Could you check a few things on this model? Use its own coordinates, in mm. A direction names the side the tool comes from. Give positions to 0.01 mm unless a question says otherwise; leave off trailing zeros. Write each loop counter-clockwise with the first axis right and the second up, starting at its lowest first coordinate (ties: lowest second). Pieces come first, ordered by that corner, then holes. Notation, with made-up numbers: M -12.75,59 L 36.25,59 A31 cw 36.25,90 Z; hole C 56,-14.75 d1. An arc over 180 degrees is marked long. Answer as a JSON object with one key per item and string values. Group by question number.
```python
from build123d import *

# Parameters (mm, degrees)
SKETCH1_W           = 100
SKETCH1_H           = 65
BOSS_EXTRUDE1_DEPTH = 35
SKETCH4_W           = 60
SKETCH4_H           = 30
CUT_EXTRUDE1_DEPTH  = 6
SKETCH5_W           = 60
SKETCH5_H           = 35
CUT_EXTRUDE2_DEPTH  = 70.14658343


with BuildPart() as part:
    # Sketch1 → Boss-Extrude1 (new body)
    with BuildSketch(Plane(origin=(0, 0, 0), x_dir=(0, 0, -1), z_dir=(1, 0, 0))):
        Rectangle(SKETCH1_W, SKETCH1_H)
    extrude(amount=BOSS_EXTRUDE1_DEPTH)

    # Sketch4 → Cut-Extrude1 (cut)
    with BuildSketch(Plane(origin=(35, 0, 0), x_dir=(0, 0, -1), z_dir=(1, 0, 0))):
        with Locations((20, -17.5)):
            Rectangle(SKETCH4_W, SKETCH4_H)
    extrude(amount=-CUT_EXTRUDE1_DEPTH, mode=Mode.SUBTRACT)

    # Sketch5 → Cut-Extrude2 (cut, through all)
    with BuildSketch(Plane(origin=(35, 0, 0), x_dir=(0, 0, -1), z_dir=(1, 0, 0))):
        with Locations((20, 15)):
            Rectangle(SKETCH5_W, SKETCH5_H)
    extrude(amount=-CUT_EXTRUDE2_DEPTH, mode=Mode.SUBTRACT)


solid = part.part
```
1) If we section it at C-C, the plane z = -27: List the corners of the cut face in (x, y) for me.
2) If we section it at D-D, the plane x = 31: List the corners of the cut face in (y, z) for me.
3) Please list where these lines run through material, in increasing order: line 1 along Z through (x, y) = (23.5, 23); line 2 along Y through (x, z) = (28.5, 4); line 3 along X through (y, z) = (-7.5, -28.5). Write a range as from..to.
4) If we section it at A-A, the plane x = 11.5: List the corners of the cut face in (y, z) for me, plus the area to 3 significant figures.
5) I'm going to push flat-ended pins straight in: pin 1 (14.5 mm diameter, centred on x = 21.5, z = -26, fed in from +Y); pin 2 (2 mm diameter, centred on y = 14, z = 14.5, fed in from -X); pin 3 (5 mm diameter, centred on y = -4, z = -28.5, fed in from +X). Where does each tip first touch, or does it pass through?
6) For faces 1 (the flat face through (15, -2.5, -20)), 2 (the flat face through (29, -17, -20)), 3 (the flat face through (35, 0, 30)), which set-ups out of +Z, -Z, +X, -X, +Y, -Y let a thin tool reach every point of the face, with its end or its side?
7) If we section it at B-B, the plane y = -6.5: List the corners of the cut face in (x, z) for me, plus the area to 3 significant figures.
Taken from the geometry:
{
 "1": {"outline": "M 0,-32.5 L 29,-32.5 L 29,-2.5 L 0,-2.5 Z"},
 "2": {"outline": "M -32.5,10 L 32.5,10 L 32.5,50 L -32.5,50 Z"},
 "3": {"line 1": "10..50", "line 2": "-32.5..-2.5", "line 3": "0..29"},
 "4": {"outline": "M -32.5,-50 L -2.5,-50 L -2.5,10 L 32.5,10 L 32.5,50 L -32.5,50 Z", "area": "4,400 mm²"},
 "5": {"pin 1": "y = -2.5", "pin 2": "x = 0", "pin 3": "x = 29"},
 "6": {"face 1": "-Z, +X, -X, +Y", "face 2": "-Z, +X, +Y, -Y", "face 3": "+Z, -Z, +X, +Y, -Y"},
 "7": {"outline": "M 0,-50 L 29,-50 L 29,10 L 35,10 L 35,50 L 0,50 Z", "area": "3,140 mm²"}
}
